Autodesk Fusion 360 part; units mm, degrees
sketch "Sketch1" plane through (0, 0, 0) normal (0, 0, 1) x (1, 0, 0)
  line L0 (2, 0) -> (162, 0)
  line L1 (164, 2) -> (164, 172)
  line L2 (162, 174) -> (2, 174)
  line L3 (0, 172) -> (0, 2)
  arc A0 (2, 174) -> (0, 172) centre (2, 172) ccw
  arc A1 (164, 172) -> (162, 174) centre (162, 172) ccw
  arc A2 (0, 2) -> (2, 0) centre (2, 2) ccw
  arc A3 (162, 0) -> (164, 2) centre (162, 2) ccw
  point P0 (164, 0)
  point P1 (0, 174)
  dimension "d1" = 164
  dimension "d2" = 174
  dimension "d3" = 2
  dimension "d4" = 2
  dimension "d5" = 2
  dimension "d6" = 2
extrude "Extrude1" add sketch "Sketch1" along normal blind 17.5
sketch "Sketch2" plane through (0, 0, 17.5) normal (0, 0, 1) x (-1, 0, 0)
  arc A0 (-162, 0) -> (-164, -2) centre (-162, -2) ccw
  line L0 (-164, -2) -> (-164, -172)
  arc A1 (-164, -172) -> (-162, -174) centre (-162, -172) ccw
  line L1 (-162, -174) -> (-2, -174)
  arc A2 (-2, -174) -> (0, -172) centre (-2, -172) ccw
  line L2 (0, -172) -> (0, -2)
  arc A3 (0, -2) -> (-2, 0) centre (-2, -2) ccw
  line L3 (-2, 0) -> (-162, 0)
  line L4 (-1, -1) -> (-163, -1)
  line L5 (-163, -1) -> (-163, -173)
  line L6 (-163, -173) -> (-1, -173)
  line L7 (-1, -173) -> (-1, -1)
  dimension "d9" = 162
  dimension "d10" = 172
  dimension "d11" = 1
  dimension "d12" = 1
extrude "Extrude2" cut sketch "Sketch2" against normal blind 5 contours L4 L5 L6 L7
sketch "Sketch3" plane through (0, 0, 12.5) normal (0, 0, 1) x (-1, 0, 0)
  line L0 (-1, -173) -> (-1, -1)
  line L1 (-1, -1) -> (-163, -1)
  line L2 (-163, -1) -> (-163, -173)
  line L3 (-163, -173) -> (-1, -173)
  line L4 (-2, -172) -> (-162, -172)
  line L5 (-162, -172) -> (-162, -2)
  line L6 (-162, -2) -> (-2, -2)
  line L7 (-2, -2) -> (-2, -172)
  dimension "d15" = 160
  dimension "d16" = 170
  dimension "d17" = 1
  dimension "d18" = 1
extrude "Extrude3" add sketch "Sketch3" along normal blind 3.4 contours L4 L5 L6 L7
sketch "Sketch5" plane through (0, 0, 15.9) normal (0, 0, 1) x (-1, 0, 0)
  line L0 (-2, -2) -> (-162, -2)
  line L1 (-162, -2) -> (-162, -172)
  line L2 (-162, -172) -> (-2, -172)
  line L3 (-2, -172) -> (-2, -2)
  line L4 (-3, -171) -> (-161, -171)
  line L5 (-161, -171) -> (-161, -3)
  line L6 (-161, -3) -> (-3, -3)
  line L7 (-3, -3) -> (-3, -171)
  dimension "d27" = 158
  dimension "d28" = 168
  dimension "d29" = 1
  dimension "d30" = 1
extrude "Extrude5" cut sketch "Sketch5" against normal blind 13.4 contours L4 L5 L6 L7
sketch "Sketch6" plane through (0, 0, 2.5) normal (0, 0, 1) x (-1, 0, 0)
  line L0 (-3, -3) -> (-161, -3)
  line L1 (-161, -3) -> (-161, -171)
  line L2 (-161, -171) -> (-3, -171)
  line L3 (-3, -171) -> (-3, -3)
  line L4 (-7.765, -168.031) -> (-64.965, -168.031)
  line L5 (-64.965, -168.031) -> (-64.965, -106.731)
  line L6 (-64.965, -106.731) -> (-7.765, -106.731)
  line L7 (-7.765, -106.731) -> (-7.765, -168.031)
  line L8 (0, -172) -> (0, -2)
  line L9 (-162, -174) -> (-2, -174)
  dimension "d33" = 57.2
  dimension "d34" = 61.3
  dimension "d35" = 7.765
  dimension "d36" = 5.969
extrude "Extrude6" cut sketch "Sketch6" against normal blind 2.5 contours L4 L5 L6 L7
fillet "Fillet1" radius 2 8 edges at (163.4142, 173.4142, 0) (82, 174, 0) (0.5858, 173.4142, 0) (0, 87, 0) (0.5858, 0.5858, 0) (82, 0, 0) (163.4142, 0.5858, 0) (164, 87, 0)
Source: CAD feature listing. Evaluate the final solid. Frame: model axes, mm. A direction names the side the tool comes from. Give positions to 0.01 mm unless a question says otherwise; leave off trailing zeros. Write each loop counter-clockwise with the first axis right and the second up, starting at its lowest first coordinate (ties: lowest second). Pieces come first, ordered by that corner, then holes.
1. Section query B-B (y = 131). Return the cut outline in (x, z) (3 decimals).
2. Section query C-C (z = 7.5). Return the cut outline in (x, y).
3. First-contact query: pin 1 (10.5 mm diameter, centred on y = 88, z = 8.5, fed in from -X); pin 2 (4 mm diameter, centred on x = 121.5, y = 119.5, fed in from +Z); pin 3 (1.2 mm diameter, centred on y = 122.5, z = 1, fed in from +X). Flat tips, straight axial feed; report the tip coordinate or a pass-through.
4. Section query A-A (x = 42.5). Return the cut outline in (y, z), then the cut area to 3 significant figures.
5. Pull-direction query (Y, two-part tool) for faces 1 (the face through (81, 0, 10)), 2 (the face through (3, 86, 9)), 3 (the face through (83, 174, 10)); classes: +Y half, -Y half, draft (parallel to the pull), parting line (faces both ways), or undercut.
6. Access query for faces 4 (the face through (0, 88, 10)), 5 (the face through (81, 171, 9)). Directions: +Z, -Z, +X, -X, +Y, -Y. A direction counts if a zero-diameter tool reaches every point of the face in a straight line with its end or side. Return the directions, or none.
7. Section query D-D (x = 145). Return the cut outline in (y, z), then the cut area to 3 significant figures.
8. Material intervals for line 1 along Y through (x, z) = (89, 4.75); line 2 along Y through (x, z) = (148.5, 15.25); line 3 along X through (y, z) = (101.5, 3.5), sorted ascending.
Output values:
1. outline: (0, 2) arc R2 ccw to (2, 0) - (7.765, 0) - (7.765, 2.5) - (3, 2.5) - (3, 15.9) - (2, 15.9) - (2, 12.5) - (1, 12.5) - (1, 17.5) - (0, 17.5) - close; (64.965, 0) - (162, 0) arc R2 ccw to (164, 2) - (164, 17.5) - (163, 17.5) - (163, 12.5) - (162, 12.5) - (162, 15.9) - (161, 15.9) - (161, 2.5) - (64.965, 2.5) - close
2. outline: (0, 2) arc R2 ccw to (2, 0) - (162, 0) arc R2 ccw to (164, 2) - (164, 172) arc R2 ccw to (162, 174) - (2, 174) arc R2 ccw to (0, 172) - close; hole (3, 3) - (161, 3) - (161, 171) - (3, 171) - close
3. pin 1: stops at x = 0
3. pin 2: stops at z = 2.5
3. pin 3: stops at x = 163.96
4. outline: (0, 2) arc R2 ccw to (2, 0) - (106.73, 0) - (106.73, 2.5) - (3, 2.5) - (3, 15.9) - (2, 15.9) - (2, 12.5) - (1, 12.5) - (1, 17.5) - (0, 17.5) - close; (168.03, 0) - (172, 0) arc R2 ccw to (174, 2) - (174, 17.5) - (173, 17.5) - (173, 12.5) - (172, 12.5) - (172, 15.9) - (171, 15.9) - (171, 2.5) - (168.03, 2.5) - close
4. area: 357 mm2
5. face 1: -Y half
5. face 2: undercut
5. face 3: +Y half
6. face 4: +Z, -Z, -X, +Y, -Y
6. face 5: +Z
7. outline: (0, 2) arc R2 ccw to (2, 0) - (172, 0) arc R2 ccw to (174, 2) - (174, 17.5) - (173, 17.5) - (173, 12.5) - (172, 12.5) - (172, 15.9) - (171, 15.9) - (171, 2.5) - (3, 2.5) - (3, 15.9) - (2, 15.9) - (2, 12.5) - (1, 12.5) - (1, 17.5) - (0, 17.5) - close
7. area: 510 mm2
8. line 1: y = 0 to 3, 171 to 174
8. line 2: y = 0 to 1, 2 to 3, 171 to 172, 173 to 174
8. line 3: x = 0 to 3, 161 to 164
